from build123d import *

# Parameters (mm, degrees)
F0_W      = 753
F0_H      = 730
F1_DEPTH  = 5
F2_W      = 551
F2_H      = 330
F2_W_2    = 543
F2_H_2    = 320
F3_DEPTH  = 500
F4_W      = 10
F4_H      = 30
F5_DEPTH  = 551
F6_W      = 5
F6_H      = 200
F7_DEPTH  = 490
F10_DEPTH = 546.401
F13_DEPTH = 5.001
F15_DEPTH = 30
F16_W     = 390
F16_H     = 320
F17_DEPTH = 30
F18_W     = 70
F18_H     = 130
F19_DEPTH = 5
F20_W     = 95
F20_H     = 310
F21_DEPTH = 5
F22_W     = 25
F22_H     = 25
F23_DEPTH = 200
F25_DEPTH = 175
F27_R     = 10
F28_DEPTH = 25


# Not quite as in the source:
# - a fillet or chamfer that OpenCascade refuses, or shapes differently, is made with other operations: its cross-section is extruded or revolved along the edge and cut away or added


with BuildPart() as f1:
    # F0 (on Front) → F1 (new body)
    with BuildSketch(Plane.XZ):
        Rectangle(F0_W, F0_H)
    extrude(amount=F1_DEPTH)

    # F2 (on face) → F3 (join)
    with BuildSketch(Plane.XZ.offset(5)):
        with Locations((-0.5, 0)):
            Rectangle(F2_W, F2_H)
        with Locations((-0.5, 0)):
            Rectangle(F2_W_2, F2_H_2, mode=Mode.SUBTRACT)
    extrude(amount=F3_DEPTH)

    # F4 (on face) → F5 (join, through all)
    with BuildSketch(Plane(origin=(-276, 0, 0), x_dir=(0, -1, 0), z_dir=(-1, 0, 0))):
        with Locations((500, 180)):
            Rectangle(F4_W, F4_H)
        with Locations((500, -180)):
            Rectangle(F4_W, F4_H)
    extrude(amount=-F5_DEPTH)

    # F6 (on face) → F7 (join, through all)
    with BuildSketch(Plane.XZ.offset(5)):
        with Locations((164.4, 265)):
            Rectangle(F6_W, F6_H)
        with Locations((53.8, 265)):
            Rectangle(F6_W, F6_H)
        with Locations((-56.8, 265)):
            Rectangle(F6_W, F6_H)
        with Locations((-167.4, 265)):
            Rectangle(F6_W, F6_H)
        with Locations((164.4, -265)):
            Rectangle(F6_W, F6_H)
        with Locations((53.8, -265)):
            Rectangle(F6_W, F6_H)
        with Locations((-56.8, -265)):
            Rectangle(F6_W, F6_H)
        with Locations((-167.4, -265)):
            Rectangle(F6_W, F6_H)
    extrude(amount=F7_DEPTH)

    # F8 (on face) + F9 (on face) → F10 (cut, through all)
    with BuildSketch(Plane(origin=(-169.9, 0, 0), x_dir=(0, -1, 0), z_dir=(-1, 0, 0))):
        Polygon((5, 365), (495, 195), (495, 365), align=None)
    with BuildSketch(Plane(origin=(-169.9, 0, 0), x_dir=(0, -1, 0), z_dir=(-1, 0, 0))):
        Polygon((495, -365), (495, -195), (5, -365), align=None)
    extrude(amount=-F10_DEPTH, mode=Mode.SUBTRACT)

    # F11 (on face) + F12 (on face) → F13 (cut, through all)
    with BuildSketch(Plane.XZ.offset(5)):
        Polygon((275, -165), (166.9, -365), (376.5, -365), (376.5, 365), (166.9, 365), (275, 165), align=None)
    with BuildSketch(Plane.XZ.offset(5)):
        Polygon((-376.5, -365), (-169.9, -365), (-276, -165), (-276, 165), (-169.9, 365), (-376.5, 365), align=None)
    extrude(amount=-F13_DEPTH, mode=Mode.SUBTRACT)

    # F14 (on face) → F15 (join)
    with BuildSketch(Plane.YZ.offset(275)):
        Polygon((-5, -165), (0, -165), (0, 165), (-5, 165), (-400, 165), (-400, -165), align=None)
    extrude(amount=F15_DEPTH)

    # F16 (on face) → F17 (cut)
    with BuildSketch(Plane(origin=(271, 0, 0), x_dir=(0, -1, 0), z_dir=(-1, 0, 0))):
        with Locations((200, 0)):
            Rectangle(F16_W, F16_H)
    extrude(amount=-F17_DEPTH, mode=Mode.SUBTRACT)

    # F18 (on face) → F19 (cut)
    with BuildSketch(Plane.YZ.offset(305)):
        with BuildLine():
            ThreePointArc((-165, 65), (-230, 0), (-165, -65))
            Line((-165, -65), (-165, 65))
        make_face()
        with Locations((-130, 0)):
            Rectangle(F18_W, F18_H)
        with BuildLine():
            Line((-95, 65), (-95, -65))
            ThreePointArc((-95, -65), (-30, 0), (-95, 65))
        make_face()
    extrude(amount=-F19_DEPTH, mode=Mode.SUBTRACT)

    # F20 (on face) → F21 (cut)
    with BuildSketch(Plane(origin=(-276, 0, 0), x_dir=(0, -1, 0), z_dir=(-1, 0, 0))):
        with Locations((447.5, 0)):
            Rectangle(F20_W, F20_H)
    extrude(amount=-F21_DEPTH, mode=Mode.SUBTRACT)

    # F22 (on face) → F23 (join)
    with BuildSketch(Plane.XZ.offset(5)):
        with Locations((212.5, 0)):
            Rectangle(F22_W, F22_H)
    extrude(amount=F23_DEPTH)

    # F24 (on face) → F25 (join)
    with BuildSketch(Plane.YZ.offset(225)):
        with BuildLine():
            ThreePointArc((-192.5, -12.5), (-183.6611652352, -8.8388347648), (-180, 0))
            ThreePointArc((-180, 0), (-183.6611652352, 8.8388347648), (-192.5, 12.5))
            ThreePointArc((-192.5, 12.5), (-201.3388347648, 8.8388347648), (-205, 0))
            ThreePointArc((-205, 0), (-201.3388347648, -8.8388347648), (-192.5, -12.5))
        make_face()
    extrude(amount=F25_DEPTH)

    # F26: chamfer of 1.1 on 1 edges, made by hand

    # F26_s1 → F26_t2 (revolve, cut)
    with BuildSketch(Plane.XZ.offset(192.5)):
        Polygon((398.9, 12.5), (400, 11.4), (400, 12.5), align=None)
    revolve(axis=Axis((400, -192.5, 0), (-1, 0, 0)), mode=Mode.SUBTRACT)

    # F27 (on face) → F28 (cut)
    with BuildSketch(Plane.XZ.offset(505)):
        with Locations((109.1, 177.5)):
            Circle(F27_R)
        with Locations((-112.1, 177.5)):
            Circle(F27_R)
        with Locations((-112.1, -177.5)):
            Circle(F27_R)
        with Locations((109.1, -177.5)):
            Circle(F27_R)
    extrude(amount=-F28_DEPTH, mode=Mode.SUBTRACT)


solid = f1.part
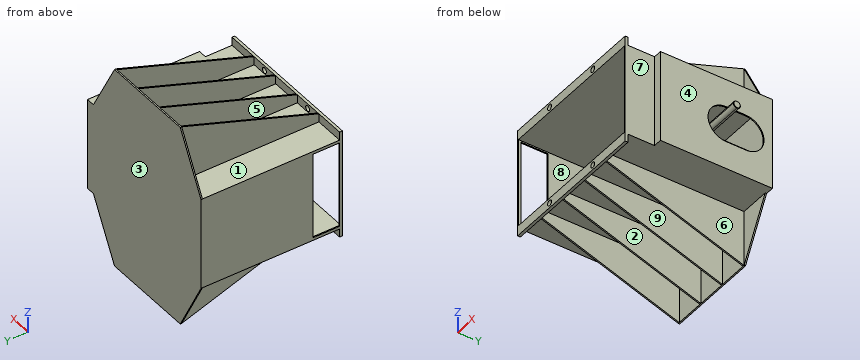
Read the model definition and answer for the solid it produces. Units are mm, in the model's axes. Face numbers are marked on the shaded views. A direction names the side the tool comes from. Give positions to 0.01 mm unless a question says otherwise; leave off trailing zeros. Write each loop counter-clockwise with the first axis right and the second up, starting at its lowest first coordinate (ties: lowest second). Pieces come first, ordered by that corner, then holes. Notation, with made-up numbers: (-6.5, 11) -> (23.5, 11) arc R27 cw to (23.5, 45) -> close; hole circle Ø7 at (38, 12.5). An arc over 180 degrees is marked (long way). Answer as a JSON object with one key per item and string values. Group by question number.
1) Each of these flat-tipped pins is pushed along its axis until it touches: P1, Ø4, axis at x = 153.5, z = 139, coming from the -Y side; P2, Ø2, axis at x = 122, y = -402.5, coming from the -Z side; P3, Ø5, axis at x = -61, y = -68, coming from the -Z side; P4, Ø24, axis at x = 106.5, z = -187.5, coming from the +Y side. Where does it stop, or does it pass through?
2) The mould has two halves that part along Y. Classify the marked faces 1, 2, 3 and 4: +Y half, -Y half, draft (parallel to the pull), parting line (faces both ways), or undercut.
3) Find section A-A (x = 109.1). Write down the section's boundary in (y, z), and give its area (3 significant figures).
4) Consider L1, parallel to X at y = -198, z = 208.5; L2, parallel to Z at x = 109.1, y = -499; L3, parallel to X at y = -501, z = 177. Determine where each line is inside the solid, lowest interval first. Write a range as from..to.
5) A tool of negligible diameter and unlimited length cuts with its end or side. For the marked faces 5, 6, 7, 8 and 9, from which of +Z, -Z, +X, -X, +Y, -Y can it reach the whole face along a straight path? Write none if from no direction.
6) Find section B-B (z = -48). Write down the section's boundary in (x, y), and give its area (3 significant figures).
7) Find section D-D (x = -154.5). Write down the section's boundary in (y, z), and give its area (3 significant figures).
Values follow:
{
 "1": {"P1": "stops at y = -5", "P2": "stops at z = -165", "P3": "stops at z = -343.78", "P4": "stops at y = 0"},
 "2": {"face 1": "undercut", "face 2": "undercut", "face 3": "+Y half", "face 4": "draft"},
 "3": {"outline": "(-505, -195) -> (-495, -195) -> (-495, -187.5) -> (-505, -187.5) -> close; (-505, -167.5) -> (-495, -167.5) -> (-495, -165) -> (-5, -165) -> (-5, -365) -> (0, -365) -> (0, 365) -> (-5, 365) -> (-5, 165) -> (-495, 165) -> (-495, 167.5) -> (-505, 167.5) -> (-505, 160) -> (-5, 160) -> (-5, -160) -> (-505, -160) -> close; (-505, 187.5) -> (-495, 187.5) -> (-495, 195) -> (-505, 195) -> close", "area": "8,850 mm2"},
 "4": {"L1": "x = -169.9..-164.9, -59.3..-54.3, 51.3..56.3, 161.9..166.9", "L2": "z = -195..-187.5, -167.5..-160, 160..167.5, 187.5..195", "L3": "x = -276..-122.09, -102.11..99.11, 119.09..275"},
 "5": {"face 5": "+Z", "face 6": "-Z, +X", "face 7": "+Z, -Z, +X, -Y", "face 8": "-Y", "face 9": "-Z"},
 "6": {"outline": "(-276, -505) -> (-272, -505) -> (-272, -495) -> (-276, -495) -> close; (-276, -400) -> (-272, -400) -> (-272, -5) -> (301, -5) -> (301, -51.17) -> (305, -51.17) -> (305, 0) -> (-276, 0) -> close; (271, -505) -> (275, -505) -> (275, -400) -> (305, -400) -> (305, -208.83) -> (301, -208.83) -> (301, -395) -> (271, -395) -> close", "area": "6,040 mm2"},
 "7": {"outline": "(-505, -195) -> (-495, -195) -> (-495, -165) -> (-5, -165) -> (-5, -365) -> (0, -365) -> (0, 365) -> (-5, 365) -> (-5, 165) -> (-495, 165) -> (-495, 195) -> (-505, 195) -> (-505, 160) -> (-5, 160) -> (-5, -160) -> (-505, -160) -> close", "area": "9,250 mm2"}
}
